```python
from build123d import *


with BuildPart() as part:
    # Sketch1 → Revolve1 (revolve)
    with BuildSketch(Plane(origin=(0, 0, 0), x_dir=(1, 0, 0), z_dir=(0, 1, 0))):
        with BuildLine():
            Line((3.5, -4.7), (3.5, -1.5))
            ThreePointArc((3.5, -1.5), (3.646446609, -1.146446609), (4, -1))
            Line((4, -1), (5.5, -1))
            Line((5.5, -1), (5.5, 0))
            Line((5.5, 0), (2.5, 0))
            Line((2.5, 0), (2.5, -5))
            Line((2.5, -5), (3.326794919, -5))
            Line((3.326794919, -5), (3.5, -4.7))
        make_face()
    revolve(axis=Axis((0, 0, 0), (0, 0, 1)))


solid = part.part
```
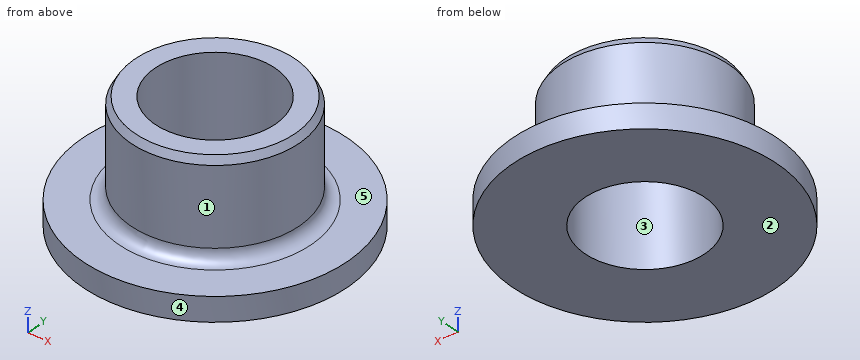
Part model, mm, in its own coordinate system. Face numbers are marked on the shaded views. A direction names the side the tool comes from. Give positions to 0.01 mm unless a question says otherwise; leave off trailing zeros. Write each loop counter-clockwise with the first axis right and the second up, starting at its lowest first coordinate (ties: lowest second). Pieces come first, ordered by that corner, then holes. Notation, with made-up numbers: (28.25, -16) -> (63.25, -16) arc R20 cw to (63.25, 2) -> close; hole circle Ø11 at (4, 1). An arc over 180 degrees is marked (long way). Put each result on its own line as item: value. Start each with the question number.
Item 1: Which spindle directions (+Z, -Z, +X, -X, +Y, -Y) get a long thin tool onto all of the face, cutting with end or side? Do the marked faces 1 and 2. Say none if no direction does.
Item 2: Pin check, flat tip, straight feed: pin 1 Ø4.5 at (x, y) = (0, 0) entering from +Z. Stop position of the tip, or through.
Item 3: Cut at D-D (x = -4.5). List the corners of the cut face in (y, z), then the cut area to 3 significant figures.
Item 4: Cut at A-A (y = 0). List the corners of the cut face in (x, z).
Item 5: Pull direction Y, two halves, no side cores. Call the marked faces 3, 4 and 5: pulls with the +Y half, pulls with the -Y half, needs draft (parallel to the pull), parting line crosses it, or undercut.
Item 6: Cut at C-C (z = 0.65). List the corners of the cut face in (x, y), then the cut area to 3 significant figures.
Item 7: Wall check: L1, parallel to Y at x = 0, z = 3.75; L2, parallel to Z at x = 3.5, y = -2.5; L3, parallel to X at y = -0.75, z = 3.1. Give the ranges that are in metal, low to high. Write a range as [from, to].
Answer list:
1. face 1: +Z
1. face 2: -Z, +X, -X, +Y, -Y
2. pin 1: passes through
3. outline: (-3.16, 0) -> (3.16, 0) -> (3.16, 1) -> (-3.16, 1) -> close
3. area: 6.32 mm2
4. outline: (-5.5, 0) -> (-2.5, 0) -> (-2.5, 5) -> (-3.33, 5) -> (-3.5, 4.7) -> (-3.5, 1.5) arc R0.5 cw to (-4, 1) -> (-5.5, 1) -> close; (2.5, 0) -> (5.5, 0) -> (5.5, 1) -> (4, 1) arc R0.5 cw to (3.5, 1.5) -> (3.5, 4.7) -> (3.33, 5) -> (2.5, 5) -> close
5. face 3: undercut
5. face 4: parting line crosses it
5. face 5: needs draft
6. outline: circle Ø11 at (0, 0); hole circle Ø5 at (0, 0)
6. area: 75.4 mm2
7. L1: y = [-3.5, -2.5], [2.5, 3.5]
7. L2: z = [0, 1]
7. L3: x = [-3.42, -2.38], [2.38, 3.42]
